```python
from build123d import *

# Parameters (mm, degrees)
SKETCH_W            = 30
SKETCH_H            = 70
PAD_DEPTH           = 3
SKETCH001_R         = 5.5
SKETCH001_R_2       = 2.5
PAD001_DEPTH        = 17.4
LINEARPATTERN_COUNT = 2
LINEARPATTERN_PITCH = 34.95
SKETCH006_R         = 5.55
POCKET_DEPTH        = 17.65
SKETCH007_R         = 5.55
POCKET003_DEPTH     = 17.65


with BuildPart() as part:
    # Sketch → Pad (new body)
    with BuildSketch(Plane.XY):
        Rectangle(SKETCH_W, SKETCH_H)
    extrude(amount=PAD_DEPTH)

    # Sketch001 (on Face1 of Pad) → Pad001 (join)
    with BuildSketch(Plane.XZ.offset(35)):
        with Locations((-15, 5.5)):
            Circle(SKETCH001_R)
        with Locations((-15, 5.5)):
            Circle(SKETCH001_R_2, mode=Mode.SUBTRACT)
    pad001 = extrude(amount=-PAD001_DEPTH)

    # LinearPattern: Pad001 ×2
    with Locations(*[(0, i * LINEARPATTERN_PITCH, 0) for i in range(1, LINEARPATTERN_COUNT)]):
        add(pad001)

    # Sketch006 (on Face12 of MultiTransform) → Pocket (cut)
    with BuildSketch(Plane(origin=(0, -17.6, 0), x_dir=(-1, 0, 0), z_dir=(0, 1, 0))):
        with Locations((15, 5.5)):
            Circle(SKETCH006_R)
    extrude(amount=POCKET_DEPTH, mode=Mode.SUBTRACT)

    # Sketch007 (on Face12 of Pocket) → Pocket003 (cut)
    with BuildSketch(Plane(origin=(0, 17.35, 0), x_dir=(-1, 0, 0), z_dir=(0, 1, 0))):
        with Locations((15, 5.5)):
            Circle(SKETCH007_R)
    extrude(amount=POCKET003_DEPTH, mode=Mode.SUBTRACT)


solid = part.part
```
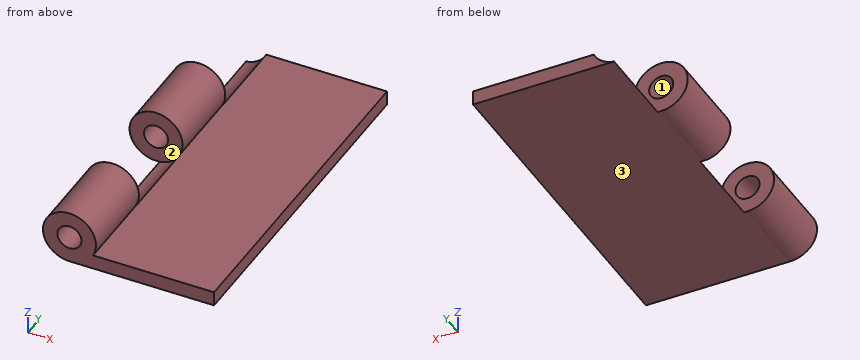
Here's how the part is built. I have some questions about the finished solid (model axes, mm). Face numbers are marked on the shaded views. Give positions to 0.01 mm unless a question says otherwise; leave off trailing zeros. Write each loop counter-clockwise with the first axis right and the second up, starting at its lowest first coordinate (ties: lowest second). Pieces come first, ordered by that corner, then holes. Notation, with made-up numbers: (24.25, 81.5) -> (33.25, 81.5) arc R29 ccw to (33.25, 117.5) -> close; hole circle Ø5 at (7, 7). An arc over 180 degrees is marked (long way). Use one line per item in the form item = value.
1) Suppose I cut it at D-D (x = 3). Please give me the cut outline in (y, z), and give its area (3 significant figures).
Verdict:
outline = (-35, 0) -> (35, 0) -> (35, 3) -> (-35, 3) -> close
area = 210 mm2
2) Suppose I cut it at A-A (z = 5.5). Please give me the cut outline in (x, y), and give its area (3 significant figures).
Verdict:
outline = (-20.5, -35) -> (-17.5, -35) -> (-17.5, -17.6) -> (-20.5, -17.6) -> close; (-20.5, 0.05) -> (-17.5, 0.05) -> (-17.5, 17.35) -> (-20.5, 17.35) -> close; (-12.5, -35) -> (-9.5, -35) -> (-9.5, -17.6) -> (-12.5, -17.6) -> close; (-12.5, 0.05) -> (-9.5, 0.05) -> (-9.5, 17.35) -> (-12.5, 17.35) -> close
area = 208 mm2
3) Suppose I cut it at C-C (x = -16.5). Please give me the cut outline in (y, z), and give its area (3 significant figures).
Verdict:
outline = (-35, 0.21) -> (-17.6, 0.21) -> (-17.6, 3.5) -> (-35, 3.5) -> close; (-35, 7.5) -> (-17.6, 7.5) -> (-17.6, 10.79) -> (-35, 10.79) -> close; (0.05, 0.21) -> (17.35, 0.21) -> (17.35, 3.5) -> (0.05, 3.5) -> close; (0.05, 7.5) -> (17.35, 7.5) -> (17.35, 10.79) -> (0.05, 10.79) -> close
area = 228 mm2
4) Suppose I cut it at B-B (y = 2). Please give me the cut outline in (x, z).
Verdict:
outline = (-15, 0) -> (15, 0) -> (15, 3) -> (-10.1, 3) arc R5.5 ccw (long way) to start; hole circle Ø5 at (-15, 5.5)
5) If I drill on L1, parallel to Z at x = -15, y = -31; L2, parallel to X at y = -23.75, z = 5.5; L3, parallel to Z at x = -4.5, y = 3, over which ranges is the centre line in solid material (lowest first)? Write a range as [from, to].
Verdict:
L1 = [0, 3], [8, 11]
L2 = [-20.5, -17.5], [-12.5, -9.5]
L3 = [0, 3]
6) We'd pull the mould along Z, two halves only. Please class the marked faces 1, 2 and 3: +Z half, -Z half, draft (parallel to the pull), parting line (faces both ways), or undercut.
Verdict:
face_1 = undercut
face_2 = draft
face_3 = -Z half
7) I'm going to push flat-ended pins straight in: pin 1 (12 mm diameter, centred on x = -5, y = -24.5, fed in from +Z); pin 2 (1.5 mm diameter, centred on y = 12.5, z = 5, fed in from +X); pin 3 (4 mm diameter, centred on y = 14, z = 9.5, fed in from -X). Where does each tip first touch, or does it pass through?
Verdict:
pin_1 = 9.27
pin_2 = -9.5
pin_3 = -20.12
